Geometry: final body of the model. Coordinates: model frame, mm. A direction names the side the tool comes from. Give positions to 0.01 mm unless a question says otherwise; leave off trailing zeros. Write each loop counter-clockwise with the first axis right and the second up, starting at its lowest first coordinate (ties: lowest second). Pieces come first, ordered by that corner, then holes.
```python
from build123d import *

# Parameters (mm, degrees)
F1_R     = 9.525
F2_DEPTH = 7.62
F4_R     = 4.0005
F5_DEPTH = 3.429
F6_R     = 3.81


with BuildPart() as f2:
    # F1 (on Front) → F2 (new body)
    with BuildSketch(Plane.XZ):
        Circle(F1_R)
    extrude(amount=F2_DEPTH)

    # F0 (on Top) → F3 (revolve, cut)
    with BuildSketch(Plane.XY):
        with BuildLine():
            Line((0, 31.75), (0, -6.35))
            ThreePointArc((0, -6.35), (19.05, 12.7), (0, 31.75))
        make_face()
    revolve(axis=Axis((0, 12.7, 0), (0, 1, 0)), mode=Mode.SUBTRACT)

    # F4 (on face) → F5 (join)
    with BuildSketch(Plane.XZ.offset(7.62)):
        Circle(F4_R)
    extrude(amount=F5_DEPTH)

    # F6
    f6_edges = [f2.edges().sort_by_distance(p)[0] for p in [
        (-9.525, -7.62, 0),
    ]]
    fillet(f6_edges, radius=F6_R)


solid = f2.part
```
Item 1: Reachability of faces 1 (the face through (2, -7.62, -4)), 2 (the face through (0, -11.049, 0)) from +Z, -Z, +X, -X, +Y, -Y: full face, straight path, thin tool, end or side. Return the list, or none.
Found:
face 1: -Y
face 2: +Z, -Z, +X, -X, -Y
Item 2: Pin query (flat end, axial travel): pin 1 Ø1 at (x, y) = (2.5, -9.5) entering from -Z; pin 2 Ø6 at (x, z) = (4, -3.5) entering from -Y; pin 3 Ø3 at (x, y) = (7, -10) entering from +Z. Return the tip coordinate at first contact, or that it passes through.
Found:
pin 1: stops at z = -3.46
pin 2: stops at y = -11.05
pin 3: passes through
Item 3: Section C-C, the plane y = -8. Return the cut outline in (x, z).
Found:
outline: circle Ø8 at (0, 0)
Item 4: Line query: L1, parallel to Z at x = 0, y = -9.25; L2, parallel to Y at x = -5, z = 1.5; L3, parallel to Y at x = -3, z = -5.5. Output: solid intervals per line, ascending.
Found:
L1: z = -4 to 4
L2: y = -7.62 to -5.62
L3: y = -7.58 to -5.29
Item 5: Section D-D, the plane y = -7. Return the cut outline in (x, z).
Found:
outline: circle Ø15.6 at (0, 0)
